from build123d import *

# Parameters (mm, degrees)
F0_W      = 124.8
F0_H      = 81
F1_DEPTH  = 15.39
F2_W      = 120.8
F2_H      = 77
F3_DEPTH  = 13.39
F4_W      = 124.8
F4_H      = 3
F5_DEPTH  = 1.15
F6_W      = 124.8
F6_H      = 3
F7_DEPTH  = 1.15
F8_W      = 78.7
F8_H      = 3
F9_DEPTH  = 1.15
F10_W     = 78.7
F10_H     = 3
F11_DEPTH = 1.15
F12_W     = 10
F12_H     = 10
F13_DEPTH = 11.82
F14_W     = 10
F14_H     = 10
F15_DEPTH = 11.82
F16_W     = 10
F16_H     = 10
F17_DEPTH = 11.82
F18_W     = 10
F18_H     = 10
F19_DEPTH = 11.82
F20_R     = 1.5
F21_DEPTH = 11.82
F22_R     = 1.5
F23_DEPTH = 11.82
F24_R     = 1.5
F25_DEPTH = 11.82
F26_R     = 1.5
F27_DEPTH = 11.82


with BuildPart() as f1:
    # F0 (on Top) → F1 (new body)
    with BuildSketch(Plane.XY):
        Rectangle(F0_W, F0_H)
    extrude(amount=F1_DEPTH)

    # F2 (on face) → F3 (cut)
    with BuildSketch(Plane.XY.offset(15.39)):
        Rectangle(F2_W, F2_H)
    extrude(amount=-F3_DEPTH, mode=Mode.SUBTRACT)

    # F4 (on face) → F5 (cut)
    with BuildSketch(Plane(origin=(0, 40.5, 0), x_dir=(-1, 0, 0), z_dir=(0, 1, 0))):
        with Locations((0, 13.89)):
            Rectangle(F4_W, F4_H)
    extrude(amount=-F5_DEPTH, mode=Mode.SUBTRACT)

    # F6 (on face) → F7 (cut)
    with BuildSketch(Plane.XZ.offset(40.5)):
        with Locations((0, 13.89)):
            Rectangle(F6_W, F6_H)
    extrude(amount=-F7_DEPTH, mode=Mode.SUBTRACT)

    # F8 (on face) → F9 (cut)
    with BuildSketch(Plane(origin=(-62.4, 0, 0), x_dir=(0, -1, 0), z_dir=(-1, 0, 0))):
        with Locations((0, 13.89)):
            Rectangle(F8_W, F8_H)
    extrude(amount=-F9_DEPTH, mode=Mode.SUBTRACT)

    # F10 (on face) → F11 (cut)
    with BuildSketch(Plane.YZ.offset(62.4)):
        with Locations((0, 13.89)):
            Rectangle(F10_W, F10_H)
    extrude(amount=-F11_DEPTH, mode=Mode.SUBTRACT)

    # F12 (on face) → F13 (join)
    with BuildSketch(Plane.XY.offset(2)):
        with Locations((-55.4, 33.5)):
            Rectangle(F12_W, F12_H)
    extrude(amount=F13_DEPTH)

    # F14 (on face) → F15 (join)
    with BuildSketch(Plane.XY.offset(2)):
        with Locations((-55.4, -33.5)):
            Rectangle(F14_W, F14_H)
    extrude(amount=F15_DEPTH)

    # F16 (on face) → F17 (join)
    with BuildSketch(Plane.XY.offset(2)):
        with Locations((55.4, -33.5)):
            Rectangle(F16_W, F16_H)
    extrude(amount=F17_DEPTH)

    # F18 (on face) → F19 (join)
    with BuildSketch(Plane.XY.offset(2)):
        with Locations((55.4, 33.5)):
            Rectangle(F18_W, F18_H)
    extrude(amount=F19_DEPTH)

    # F20 (on face) → F21 (cut)
    with BuildSketch(Plane.XY.offset(13.82)):
        with Locations((-55, 33.5)):
            Circle(F20_R)
    extrude(amount=-F21_DEPTH, mode=Mode.SUBTRACT)

    # F22 (on face) → F23 (cut)
    with BuildSketch(Plane.XY.offset(13.82)):
        with Locations((-55, -33.5)):
            Circle(F22_R)
    extrude(amount=-F23_DEPTH, mode=Mode.SUBTRACT)

    # F24 (on face) → F25 (cut)
    with BuildSketch(Plane.XY.offset(13.82)):
        with Locations((55, -33.5)):
            Circle(F24_R)
    extrude(amount=-F25_DEPTH, mode=Mode.SUBTRACT)

    # F26 (on face) → F27 (cut)
    with BuildSketch(Plane.XY.offset(13.82)):
        with Locations((55, 33.5)):
            Circle(F26_R)
    extrude(amount=-F27_DEPTH, mode=Mode.SUBTRACT)


solid = f1.part
Geometry check sheet. Reference: the model listing, model coordinates, mm. A direction names the side the tool comes from. Give positions to 0.01 mm unless a question says otherwise; leave off trailing zeros. Order: outer loops, then holes, each group sorted by start corner. A loop starts at its lowest first (then second) coordinate and runs counter-clockwise, first axis right, second up.
1. Depth check by flat-ended pin: pin 1 (5 mm diameter, centred on y = 22, z = 13.5, fed in from -X); pin 2 (5 mm diameter, centred on x = -57.5, y = -31, fed in from +Z); pin 3 (8 mm diameter, centred on x = -40.5, y = -14, fed in from +Z). Enter the tip coordinate at first touch or a pass-through.
Completed:
pin 1: stops at x = -62.4
pin 2: stops at z = 13.82
pin 3: stops at z = 2
2. Sectioned sample at C-C (y = -33.5). Record the boundary of the cut face in (x, z).
Completed:
outline: (-62.4, 0) - (62.4, 0) - (62.4, 12.39) - (61.25, 12.39) - (61.25, 15.39) - (60.4, 15.39) - (60.4, 13.82) - (56.5, 13.82) - (56.5, 2) - (53.5, 2) - (53.5, 13.82) - (50.4, 13.82) - (50.4, 2) - (-50.4, 2) - (-50.4, 13.82) - (-53.5, 13.82) - (-53.5, 2) - (-56.5, 2) - (-56.5, 13.82) - (-60.4, 13.82) - (-60.4, 15.39) - (-61.25, 15.39) - (-61.25, 12.39) - (-62.4, 12.39) - close
3. Sectioned sample at A-A (z = 6.5). Record the boundary of the cut face in (x, y).
Completed:
outline: (-62.4, -40.5) - (62.4, -40.5) - (62.4, 40.5) - (-62.4, 40.5) - close; hole (-60.4, -28.5) - (-50.4, -28.5) - (-50.4, -38.5) - (50.4, -38.5) - (50.4, -28.5) - (60.4, -28.5) - (60.4, 28.5) - (50.4, 28.5) - (50.4, 38.5) - (-50.4, 38.5) - (-50.4, 28.5) - (-60.4, 28.5) - close; hole circle Ø3 at (-55, -33.5); hole circle Ø3 at (-55, 33.5); hole circle Ø3 at (55, -33.5); hole circle Ø3 at (55, 33.5)
4. Scan lines: line 1 (Y direction, x = 55, z = 7); line 2 (X direction, y = 13, z = 10.75); line 3 (X direction, y = -30.5, z = 2.25). Record each from-to range of solid material in increasing order.
Completed:
line 1: y = -40.5 to -35, -32 to -28.5, 28.5 to 32, 35 to 40.5
line 2: x = -62.4 to -60.4, 60.4 to 62.4
line 3: x = -62.4 to -50.4, 50.4 to 62.4
5. Sectioned sample at B-B (x = -4.5). Record the boundary of the cut face in (y, z).
Completed:
outline: (-40.5, 0) - (40.5, 0) - (40.5, 12.39) - (39.35, 12.39) - (39.35, 15.39) - (38.5, 15.39) - (38.5, 2) - (-38.5, 2) - (-38.5, 15.39) - (-39.35, 15.39) - (-39.35, 12.39) - (-40.5, 12.39) - close
6. Draft check along Y on faces 1 (the face through (-50.4, -34, 8)), 2 (the face through (-1, 1, 0)), 3 (the face through (-1, -40.5, 6)). Enter one of: pulls with the +Y half, pulls with the -Y half, needs draft (parallel to the pull), parting line crosses it, or undercut.
Completed:
face 1: undercut
face 2: needs draft
face 3: pulls with the -Y half
7. Sectioned sample at D-D (y = 22). Record the boundary of the cut face in (x, z), then the cut area to 3 significant figures.
Completed:
outline: (-62.4, 0) - (62.4, 0) - (62.4, 12.39) - (61.25, 12.39) - (61.25, 15.39) - (60.4, 15.39) - (60.4, 2) - (-60.4, 2) - (-60.4, 15.39) - (-61.25, 15.39) - (-61.25, 12.39) - (-62.4, 12.39) - close
area: 296 mm2
8. Access from +Z, -Z, +X, -X, +Y, -Y to the whole of each face (thin tool, end or side, straight path). Record for faces 4 (the face through (-54.31, -34.83, 7.99)), 5 (the face through (-1, 40.5, 6)), 6 (the face through (-61.25, 1, 14)).
Completed:
face 4: +Z
face 5: +Z, -Z, +X, -X, +Y
face 6: +Z, -X, +Y, -Y
